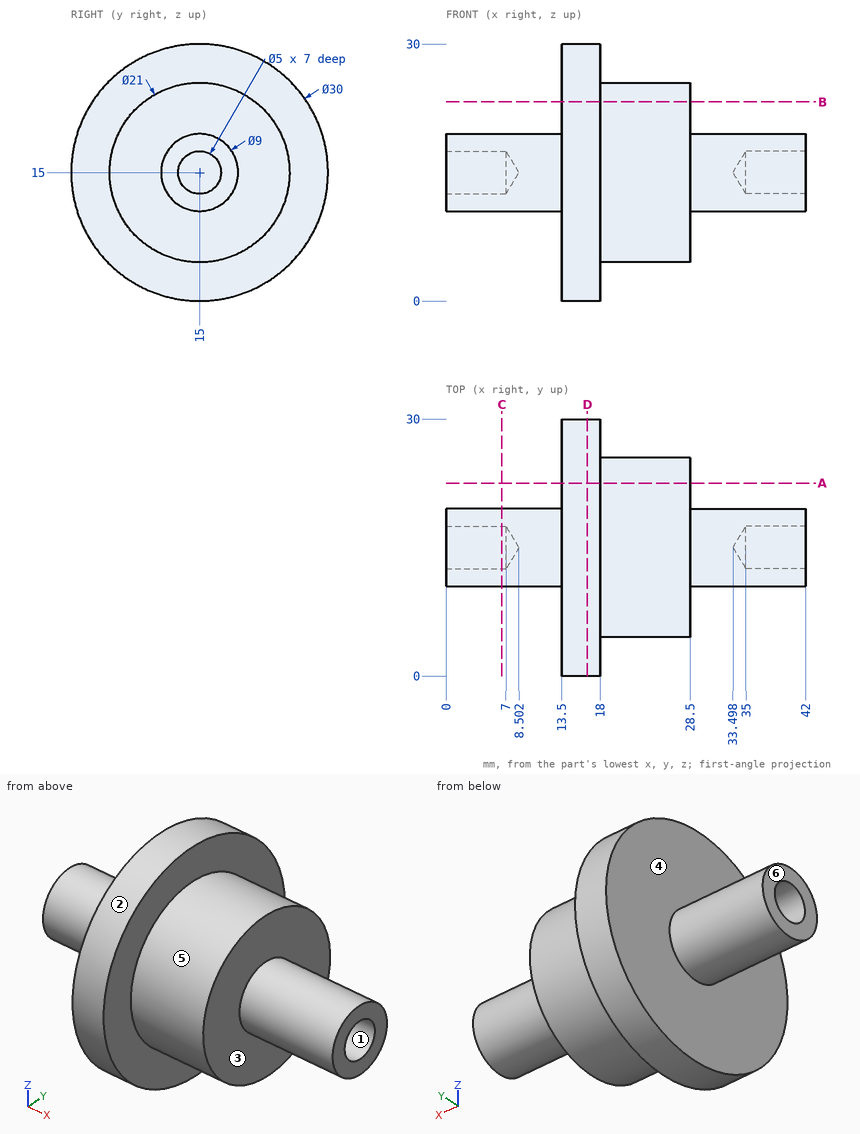
Design review of the part shown in the three views and the two pictorial views. Dimensions are in mm from the part's minimum x, y and z. A direction names the side the tool comes from. Coordinates: 2 decimals unless noted, no trailing zeros. Write each loop counter-clockwise with the first axis right and the second up, starting at its lowest first coordinate (ties: lowest second). Pieces come first, ordered by that corner, then holes.
(1) Add section D-D on x = 16.5. Give the boundary of the cut face in (y, z).
(2) Add section B-B on z = 23.25. Give the boundary of the cut face in (x, y) (1 decimal), then the cut area to 3 significant figures.
(3) Wall thickness on probe 1 along Z at (x, y) = (38.25, 15); probe 2 along X at (y, z) = (9.5, 18.5); probe 3 along Y at (x, z) = (40.5, 18.75): over which ranges is each line inside the solid? List them lowest first.
(4) Add section A-A on y = 22.5. Give the boundary of the cut face in (x, z).
(5) Add section C-C on x = 6.5. Give the boundary of the cut face in (y, z).
(6) Tool access review of the marked faces 4, 5 and 6: name each direction out of +Z, -Z, +X, -X, +Y, -Y from which nothing blocks a thin tool from reaching the whole face with its end or side.
(7) The part is to be moulded in two halves that separate along Z. For the marked faces 1, 2 and 3, say which applies: +Z half, -Z half, draft (parallel to the pull), parting line (faces both ways), or undercut.
(8) For pin 1 Ø1.5 at (x, z) = (12.5, 21.5) entering from +Y; pin 2 Ø4 at (y, z) = (17, 24) entering from -X; pin 3 Ø12 at (x, y) = (13, 22.5) entering from -Z; pin 4 Ø3 at (x, y) = (25, 15) entering from -Z, all flat-tipped, find the tip position at first contact; note any pin that passes through.
Answer sheet:
1. outline: circle Ø30 at (15, 15)
2. outline: (13.5, 2.5) - (18, 2.5) - (18, 8.5) - (28.5, 8.5) - (28.5, 21.5) - (18, 21.5) - (18, 27.5) - (13.5, 27.5) - close
2. area: 249 mm2
3. probe 1: z = 10.5 to 12.5, 17.5 to 19.5
3. probe 2: x = 13.5 to 28.5
3. probe 3: y = 12.51 to 17.49
4. outline: (13.5, 2.01) - (18, 2.01) - (18, 7.65) - (28.5, 7.65) - (28.5, 22.35) - (18, 22.35) - (18, 27.99) - (13.5, 27.99) - close
5. outline: circle Ø9 at (15, 15); hole circle Ø5 at (15, 15)
6. face 4: -X
6. face 5: +X
6. face 6: +Z, -Z, -X, +Y, -Y
7. face 1: undercut
7. face 2: parting line
7. face 3: draft
8. pin 1: passes through
8. pin 2: stops at x = 13.5
8. pin 3: stops at z = 0.08
8. pin 4: stops at z = 4.5
